from build123d import *

# Parameters (mm, degrees)
SKETCH1_W               = 215.9
SKETCH1_H               = 127
BOSS_EXTRUDE1_DEPTH     = 31.75
CUT_EXTRUDE1_START      = -12.7
CUT_EXTRUDE1_DEPTH      = 19.05
LPATTERN1_COUNT         = 2
LPATTERN1_PITCH         = 82.55
LPATTERN1_COUNT_DIR2    = 2
LPATTERN1_PITCH_DIR2    = 177.8
F_1_4_20_TAPPED_HOLE1_D = 5.1054
LPATTERN7_COUNT         = 6
LPATTERN7_PITCH         = 25.4
LPATTERN10_COUNT        = 7
LPATTERN10_PITCH        = 25.4
LPATTERN10_COUNT_DIR2   = 5
LPATTERN10_PITCH_DIR2   = 25.4


with BuildPart() as part:
    # Sketch1 → Boss-Extrude1 (new body)
    with BuildSketch(Plane.XY):
        with Locations((107.95, 63.5)):
            Rectangle(SKETCH1_W, SKETCH1_H)
    extrude(amount=BOSS_EXTRUDE1_DEPTH)

    # Sketch2 → Cut-Extrude1 (cut)
    with BuildSketch(Plane.XZ.offset(CUT_EXTRUDE1_START)):
        Polygon((13.7668, 31.75), (13.7668, 24.765), (15.4813, 24.765), (15.4813, 0), (22.6187, 0), (22.6187, 24.765), (24.3332, 24.765), (24.3332, 31.75), align=None)
    cut_extrude1 = extrude(amount=-CUT_EXTRUDE1_DEPTH, mode=Mode.SUBTRACT)

    # Sketch4 → Cut-Revolve3 (revolve, cut)
    with BuildSketch(Plane.XZ.offset(-31.75)):
        Polygon((19.05, 0), (19.05, 31.75), (13.7668, 31.75), (13.7668, 24.765), (15.4813, 24.765), (15.4813, 0), align=None)
    cut_revolve3 = revolve(axis=Axis((19.05, 31.75, 0), (0, 0, 1)), mode=Mode.SUBTRACT)

    # Sketch6 → Cut-Revolve4 (revolve, cut)
    with BuildSketch(Plane(origin=(0, 12.7, 0), x_dir=(1, 0, 0), z_dir=(0, 1, 0))):
        Polygon((19.05, 0), (19.05, -31.75), (24.3332, -31.75), (24.3332, -24.765), (22.6187, -24.765), (22.6187, 0), align=None)
    cut_revolve4 = revolve(axis=Axis((19.05, 12.7, 0), (0, 0, 1)), mode=Mode.SUBTRACT)

    # LPattern1: Cut-Extrude1, Cut-Revolve3, Cut-Revolve4 2 × 2
    with Locations(*[(j * LPATTERN1_PITCH_DIR2, i * LPATTERN1_PITCH, 0) for i in range(LPATTERN1_COUNT) for j in range(LPATTERN1_COUNT_DIR2) if (i, j) != (0, 0)]):
        add(cut_extrude1, mode=Mode.SUBTRACT)
        add(cut_revolve3, mode=Mode.SUBTRACT)
        add(cut_revolve4, mode=Mode.SUBTRACT)

    # 1/4-20 Tapped Hole1 (through all)
    with Locations(Plane.XY.offset(31.75)):
        with Locations((31.75, 12.7)):
            f_1_4_20_tapped_hole1 = Hole(F_1_4_20_TAPPED_HOLE1_D / 2)

    # Sketch14 → 1/4-20 Tapped Hole3 (revolve, cut)
    with BuildSketch(Plane(origin=(215.9, 50.8, 15.875), x_dir=(0, 0, -1), z_dir=(0, 1, 0))):
        Polygon((0, 0), (0, 33.283816902), (2.5527, 31.75), (2.5527, 0), align=None)
    f_1_4_20_tapped_hole3 = revolve(axis=Axis((222.25, 50.8, 15.875), (-1, 0, 0)), mode=Mode.SUBTRACT)

    # Sketch22 → 1/4-20 Tapped Hole5 (revolve, cut)
    with BuildSketch(Plane(origin=(171.45, 127, 15.875), x_dir=(0, 0, 1), z_dir=(1, 0, 0))):
        Polygon((0, 0), (0, 33.283816902), (2.5527, 31.75), (2.5527, 0), align=None)
    f_1_4_20_tapped_hole5 = revolve(axis=Axis((171.45, 133.35, 15.875), (0, -1, 0)), mode=Mode.SUBTRACT)

    # LPattern7: 1/4-20 Tapped Hole5 ×6
    with Locations(*[(-i * LPATTERN7_PITCH, 0, 0) for i in range(1, LPATTERN7_COUNT)]):
        add(f_1_4_20_tapped_hole5, mode=Mode.SUBTRACT)

    # LPattern10: 1_4-20 Tapped Hole1 7 × 5
    with Locations(*[(i * LPATTERN10_PITCH, j * LPATTERN10_PITCH_DIR2, 0) for i in range(LPATTERN10_COUNT) for j in range(LPATTERN10_COUNT_DIR2) if (i, j) != (0, 0)]):
        add(f_1_4_20_tapped_hole1, mode=Mode.SUBTRACT)

    # Mirror1: 1/4-20 Tapped Hole3 across plane
    add(f_1_4_20_tapped_hole3.mirror(Plane(origin=(107.95, 0, 0), x_dir=(0, 0, 1), z_dir=(1, 0, 0))), mode=Mode.SUBTRACT)

    # Mirror2: 1/4-20 Tapped Hole3 across plane
    add(f_1_4_20_tapped_hole3.mirror(Plane.ZX.offset(63.5)), mode=Mode.SUBTRACT)

    # Mirror2 copy 1 sketch → Mirror2 copy 1 (revolve, cut)
    with BuildSketch(Plane(origin=(0, 76.2, 15.875), x_dir=(0, 0, -1), z_dir=(0, -1, 0))):
        Polygon((0, 0), (0, 33.283816902), (2.5527, 31.75), (2.5527, 0), align=None)
    revolve(axis=Axis((-6.35, 76.2, 15.875), (1, 0, 0)), mode=Mode.SUBTRACT)

    # Mirror3: 1/4-20 Tapped Hole5 across plane
    add(f_1_4_20_tapped_hole5.mirror(Plane.ZX.offset(63.5)), mode=Mode.SUBTRACT)

    # Mirror3 copy 1 sketch → Mirror3 copy 1 (revolve, cut)
    with BuildSketch(Plane(origin=(146.05, 0, 15.875), x_dir=(0, 0, 1), z_dir=(1, 0, 0))):
        Polygon((0, 0), (0, -33.283816902), (2.5527, -31.75), (2.5527, 0), align=None)
    revolve(axis=Axis((146.05, -6.35, 15.875), (0, -1, 0)), mode=Mode.SUBTRACT)

    # Mirror3 copy 2 sketch → Mirror3 copy 2 (revolve, cut)
    with BuildSketch(Plane(origin=(120.65, 0, 15.875), x_dir=(0, 0, 1), z_dir=(1, 0, 0))):
        Polygon((0, 0), (0, -33.283816902), (2.5527, -31.75), (2.5527, 0), align=None)
    revolve(axis=Axis((120.65, -6.35, 15.875), (0, -1, 0)), mode=Mode.SUBTRACT)

    # Mirror3 copy 3 sketch → Mirror3 copy 3 (revolve, cut)
    with BuildSketch(Plane(origin=(95.25, 0, 15.875), x_dir=(0, 0, 1), z_dir=(1, 0, 0))):
        Polygon((0, 0), (0, -33.283816902), (2.5527, -31.75), (2.5527, 0), align=None)
    revolve(axis=Axis((95.25, -6.35, 15.875), (0, -1, 0)), mode=Mode.SUBTRACT)

    # Mirror3 copy 4 sketch → Mirror3 copy 4 (revolve, cut)
    with BuildSketch(Plane(origin=(69.85, 0, 15.875), x_dir=(0, 0, 1), z_dir=(1, 0, 0))):
        Polygon((0, 0), (0, -33.283816902), (2.5527, -31.75), (2.5527, 0), align=None)
    revolve(axis=Axis((69.85, -6.35, 15.875), (0, -1, 0)), mode=Mode.SUBTRACT)

    # Mirror3 copy 5 sketch → Mirror3 copy 5 (revolve, cut)
    with BuildSketch(Plane(origin=(44.45, 0, 15.875), x_dir=(0, 0, 1), z_dir=(1, 0, 0))):
        Polygon((0, 0), (0, -33.283816902), (2.5527, -31.75), (2.5527, 0), align=None)
    revolve(axis=Axis((44.45, -6.35, 15.875), (0, -1, 0)), mode=Mode.SUBTRACT)


solid = part.part
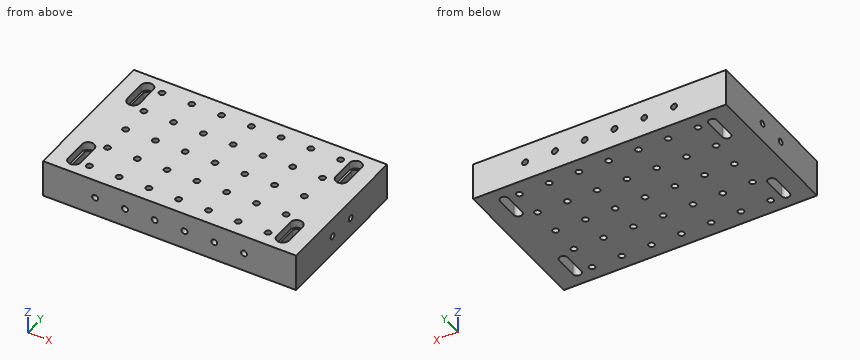
CAD build for the part. Positions are in the model's coordinates, mm. Give positions to 0.01 mm unless a question says otherwise; leave off trailing zeros. Write each loop counter-clockwise with the first axis right and the second up, starting at its lowest first coordinate (ties: lowest second). Pieces come first, ordered by that corner, then holes. Notation, with made-up numbers: (-30, -24) -> (3, -24) arc R8 ccw to (3, -9) -> close; hole circle Ø10 at (-15, -10). An arc over 180 degrees is marked (long way). Return JSON: item names as keys, results as strings.
Item 1: Band-saw the part on B-B (x = 158.75). List the corners of the cut face in (y, z).
Answer below:
{"outline": "(0, 0) -> (10.15, 0) -> (10.15, 31.75) -> (0, 31.75) -> close; (15.25, 0) -> (35.55, 0) -> (35.55, 31.75) -> (15.25, 31.75) -> close; (40.65, 0) -> (60.95, 0) -> (60.95, 31.75) -> (40.65, 31.75) -> close; (66.05, 0) -> (86.35, 0) -> (86.35, 31.75) -> (66.05, 31.75) -> close; (91.45, 0) -> (111.75, 0) -> (111.75, 31.75) -> (91.45, 31.75) -> close; (116.85, 0) -> (127, 0) -> (127, 31.75) -> (116.85, 31.75) -> close"}
Item 2: Band-saw the part on A-A (y = 104). Give the number of separate pieces and of enclosed holes in the cut face, then the cut area to 3 significant figures.
Answer below:
{"separate pieces": "3", "enclosed holes": "6", "area": "6,230 mm2"}
Item 3: Drill centre lines: probe 1 along Y at (x, z) = (107.95, 14.5); probe 2 along X at (y, z) = (26, 2). Where is each one in solid material? Low to high.
Answer below:
{"probe 1": "y = 0 to 10.15, 15.25 to 35.55, 40.65 to 60.95, 66.05 to 86.35, 91.45 to 111.75, 116.85 to 127", "probe 2": "x = 0 to 15.48, 22.62 to 193.28, 200.42 to 215.9"}
Item 4: Drop flat-ended pins along their axis: pin 1 (3 mm diameter, centred on x = 144.5, z = 10, fed in from -Y); pin 2 (4.5 mm diameter, centred on x = 57.15, y = 12.7, fed in from +Z); pin 3 (3 mm diameter, centred on x = 95.25, z = 15.875, fed in from +Y); pin 4 (4.5 mm diameter, centred on y = 76.2, z = 15.875, fed in from +X). Give the stop position or say it passes through.
Answer below:
{"pin 1": "stops at y = 0", "pin 2": "passes through", "pin 3": "stops at y = 94.62", "pin 4": "stops at x = 183.97"}
